Study the drawing (mm; zero at the part's minimum x, y, z) and answer. Coordinates: 2 decimals unless noted, no trailing zeros. Loops run counter-clockwise (first coordinate to the right, second up) from the corner with the lowest first, then second, coordinate; pieces in that order, holes last. Notation, with made-up numbers: (-36.5, -7.75) -> (-19.5, -7.75) arc R13 ccw to (-19.5, 6.25) -> close; hole circle Ø10 at (82.25, 9). An arc over 180 degrees is marked (long way). Answer in a Markdown table with one row per item.
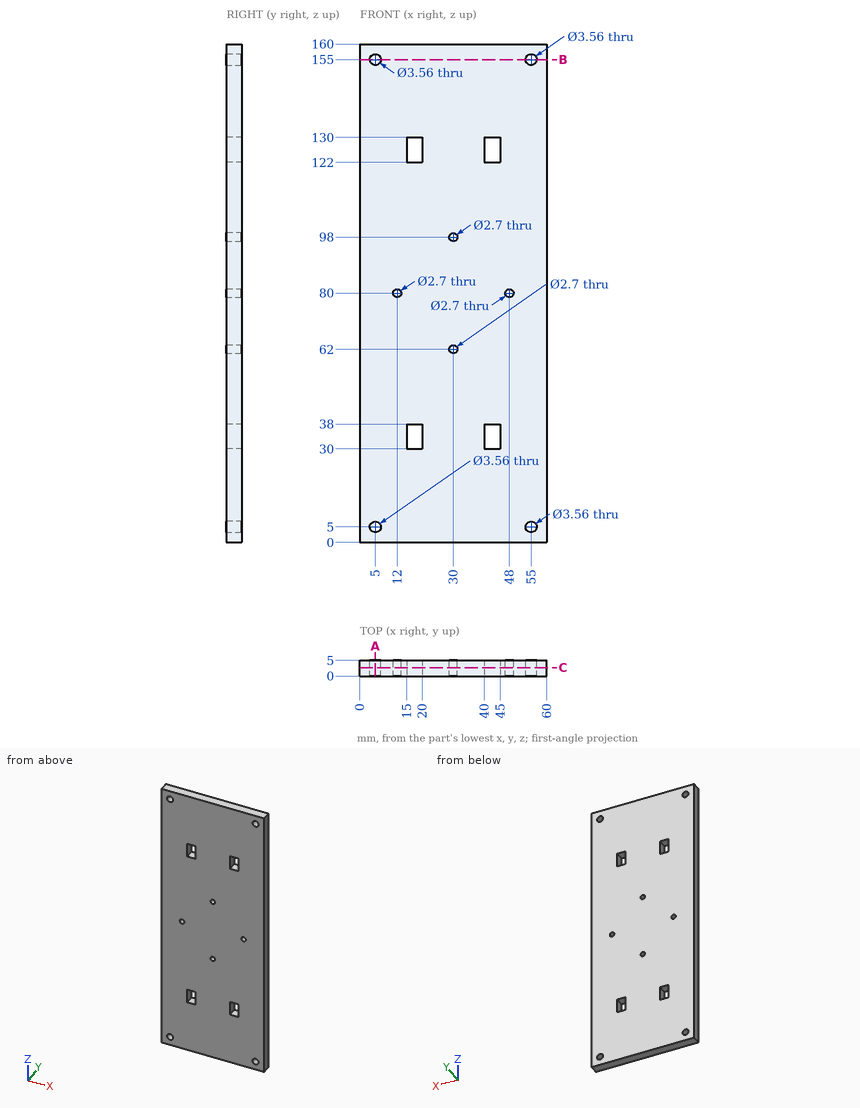
1. A cutting plane is placed at A-A on x = 5. Give the vertices of the cut face in (y, z).
A:
| item | result |
|---|---|
| outline | (0, 0) -> (5, 0) -> (5, 3.22) -> (0, 3.22) -> close; (0, 6.78) -> (5, 6.78) -> (5, 153.22) -> (0, 153.22) -> close; (0, 156.78) -> (5, 156.78) -> (5, 160) -> (0, 160) -> close |
2. A cutting plane is placed at C-C on y = 2.7. Count the separate pieces of the cut face and the enclosed holes in it, and give its area (3 significant figures).
A:
| item | result |
|---|---|
| separate pieces | 1 |
| enclosed holes | 12 |
| area | 9,380 mm2 |
3. Find the intervals of material crossed by probe 1 along X at (y, z) = (1.8, 155); probe 2 along Z at (x, y) = (18, 2.4); probe 3 along Z at (x, y) = (54.5, 0.9), in increasing order.
A:
| item | result |
|---|---|
| probe 1 | x = 0 to 3.22, 6.78 to 53.22, 56.78 to 60 |
| probe 2 | z = 0 to 30, 38 to 122, 130 to 160 |
| probe 3 | z = 0 to 3.29, 6.71 to 153.29, 156.71 to 160 |
4. A cutting plane is placed at B-B on z = 155. Give the vertices of the cut face in (x, y), and give its area (3 significant figures).
A:
| item | result |
|---|---|
| outline | (0, 0) -> (3.22, 0) -> (3.22, 5) -> (0, 5) -> close; (6.78, 0) -> (53.22, 0) -> (53.22, 5) -> (6.78, 5) -> close; (56.78, 0) -> (60, 0) -> (60, 5) -> (56.78, 5) -> close |
| area | 264 mm2 |
